from build123d import *

# Parameters (mm, degrees)
BOSS_EXTRUDE2_DEPTH     = 69.85
BOSS_EXTRUDE3_START     = 69.85
BOSS_EXTRUDE3_DEPTH     = 20.6375
BOSS_EXTRUDE4_START     = 90.4875
BOSS_EXTRUDE4_DEPTH     = 23.8125
BOSS_EXTRUDE5_START     = 69.85
BOSS_EXTRUDE5_DEPTH     = 19.05
SKETCH2_R               = 50.8
CUT_EXTRUDE1_DEPTH      = 632.689369865
SKETCH3_R               = 12.7
CUT_EXTRUDE2_DEPTH      = 38.1
CUT_EXTRUDE3_REACH      = 587.992
CUT_EXTRUDE3_END_RADIUS = 73.025
SKETCH4_R               = 7.9375


# Read off the part's stored shape, not the designer's step: Boss-Extrude4
with BuildPart() as part:
    # Sketch1 → Boss-Extrude2 (new body)
    with BuildSketch(Plane(origin=(0, 0, 0), x_dir=(0, 0, -1), z_dir=(1, 0, 0))):
        with BuildLine():
            Line((0, 381), (0, 0))
            Line((0, 0), (-82.55, 0))
            Line((-82.55, 0), (-82.55, -88.9))
            Line((-82.55, -88.9), (69.85, -88.9))
            Line((69.85, -88.9), (69.85, 0))
            Line((69.85, 0), (406.4, 0))
            Line((406.4, 0), (406.4, 117.475))
            Line((406.4, 117.475), (260.35, 117.475))
            Line((260.35, 117.475), (260.35, 111.401610843))
            Line((260.35, 111.401610843), (247.65, 111.401610843))
            Line((247.65, 111.401610843), (247.65, 117.751610843))
            ThreePointArc((247.65, 117.751610843), (181.425166335, 182.404066236), (231.775, 260.060764803))
            Line((231.775, 260.060764803), (231.775, 317.5))
            Line((231.775, 317.5), (76.2, 317.5))
            Line((76.2, 317.5), (76.2, 381))
            Line((76.2, 381), (63.5, 381))
            Line((63.5, 381), (63.5, 368.3))
            Line((63.5, 368.3), (38.1, 368.3))
            Line((38.1, 368.3), (38.1, 381))
            Line((38.1, 381), (0, 381))
        make_face()
    boss_extrude2 = extrude(amount=BOSS_EXTRUDE2_DEPTH)

    # Sketch1<4> → Boss-Extrude3 (add)
    with BuildSketch(Plane(origin=(0, 0, 0), x_dir=(0, 0, -1), z_dir=(1, 0, 0)).offset(BOSS_EXTRUDE3_START)):
        with BuildLine():
            Line((0, 381), (0, 0))
            Line((0, 0), (406.4, 0))
            Line((406.4, 0), (406.4, 190.5))
            ThreePointArc((406.4, 190.5), (388.283807472, 262.566768006), (338.242269675, 317.5))
            Line((338.242269675, 317.5), (76.2, 317.5))
            Line((76.2, 317.5), (76.2, 381))
            Line((76.2, 381), (63.5, 381))
            Line((63.5, 381), (63.5, 368.3))
            Line((63.5, 368.3), (38.1, 368.3))
            Line((38.1, 368.3), (38.1, 381))
            Line((38.1, 381), (0, 381))
        make_face()
        with BuildLine():
            Line((260.35, 117.751610843), (260.35, 111.401610843))
            Line((260.35, 111.401610843), (247.65, 111.401610843))
            Line((247.65, 111.401610843), (247.65, 117.751610843))
            ThreePointArc((247.65, 117.751610843), (254, 263.525), (260.35, 117.751610843))
        make_face(mode=Mode.SUBTRACT)
    boss_extrude3 = extrude(amount=BOSS_EXTRUDE3_DEPTH)

    # Boss-Extrude4 outline → Boss-Extrude4 (add)
    with BuildSketch(Plane(origin=(0, 0, 0), x_dir=(0, 0, -1), z_dir=(1, 0, 0)).offset(BOSS_EXTRUDE4_START)):
        Polygon((406.4, 317.5), (76.2, 317.5), (76.2, 381), (63.5, 381), (63.5, 368.3), (38.1, 368.3), (38.1, 381), (0, 381), (0, 0), (406.4, 0), align=None)
        with BuildLine():
            Line((247.65, 111.401610843), (247.65, 117.751610843))
            ThreePointArc((247.65, 117.751610843), (254, 263.525), (260.35, 117.751610843))
            Line((260.35, 117.751610843), (260.35, 111.401610843))
            Line((260.35, 111.401610843), (247.65, 111.401610843))
        make_face(mode=Mode.SUBTRACT)
    boss_extrude4 = extrude(amount=BOSS_EXTRUDE4_DEPTH)

    # Sketch1<6> → Boss-Extrude5 (add)
    with BuildSketch(Plane(origin=(0, 0, 0), x_dir=(0, 0, -1), z_dir=(1, 0, 0)).offset(BOSS_EXTRUDE5_START)):
        Polygon((69.85, 0), (0, 0), (-82.55, 0), (-82.55, -88.9), (69.85, -88.9), align=None)
    boss_extrude5 = extrude(amount=BOSS_EXTRUDE5_DEPTH)

    # Mirror2: Boss-Extrude2, Boss-Extrude3, Boss-Extrude4, Boss-Extrude5 across plane
    add(boss_extrude2.mirror(Plane(origin=(0, 0, 0), x_dir=(0, 0, 1), z_dir=(1, 0, 0))))
    add(boss_extrude3.mirror(Plane(origin=(0, 0, 0), x_dir=(0, 0, 1), z_dir=(1, 0, 0))))
    add(boss_extrude4.mirror(Plane(origin=(0, 0, 0), x_dir=(0, 0, 1), z_dir=(1, 0, 0))))
    add(boss_extrude5.mirror(Plane(origin=(0, 0, 0), x_dir=(0, 0, 1), z_dir=(1, 0, 0))))

    # Sketch2 → Cut-Extrude1 (cut, through all)
    with BuildSketch(Plane(origin=(0, 381, 0), x_dir=(1, 0, 0), z_dir=(0, 1, 0))):
        with Locations(Location((0, 0, 0), (0, 0, 270))):
            Circle(SKETCH2_R)
        with BuildLine():
            Line((-88.9, -88.9), (88.9, -88.9))
            Line((88.9, -88.9), (88.9, -6.35))
            Line((88.9, -6.35), (87.988181024, -6.35))
            ThreePointArc((87.988181024, -6.35), (83.831130216, -7.899851193), (81.703310951, -11.792857143))
            ThreePointArc((81.703310951, -11.792857143), (0, -82.55), (-81.703310951, -11.792857143))
            ThreePointArc((-81.703310951, -11.792857143), (-83.831130216, -7.899851193), (-87.988181024, -6.35))
            Line((-87.988181024, -6.35), (-88.9, -6.35))
            Line((-88.9, -6.35), (-88.9, -88.9))
        make_face()
    extrude(amount=-CUT_EXTRUDE1_DEPTH, mode=Mode.SUBTRACT)

    # Sketch3 → Cut-Extrude2 (cut)
    with BuildSketch(Plane(origin=(0, 368.3, 0), x_dir=(1, 0, 0), z_dir=(0, 1, 0))):
        with Locations(Location((-79.375, 50.8, 0), (0, 0, 270))):
            Circle(SKETCH3_R)
        with Locations(Location((79.375, 50.8, 0), (0, 0, 270))):
            Circle(SKETCH3_R)
    extrude(amount=-CUT_EXTRUDE2_DEPTH, mode=Mode.SUBTRACT)

    # Cut-Extrude3: up to this cylinder (the profile starts outside it)
    cut_extrude3_end = Plane(origin=(0, 190.5, -254), z_dir=(-1, 0, 0)) * Cylinder(CUT_EXTRUDE3_END_RADIUS, 1508.7715, mode=Mode.PRIVATE)
    # Sketch4 → Cut-Extrude3 (cut, up to the surface)
    with BuildSketch(Plane(origin=(0, 317.5, 0), x_dir=(1, 0, 0), z_dir=(0, 1, 0)), mode=Mode.PRIVATE) as cut_extrude3_sk1:
        with Locations(Location((-92.86875, 254, 0), (0, 0, 270))):
            Circle(SKETCH4_R)
    cut_extrude3_tool1 = extrude(cut_extrude3_sk1.sketch, amount=-CUT_EXTRUDE3_REACH, mode=Mode.PRIVATE) - cut_extrude3_end
    add(cut_extrude3_tool1.solids().sort_by_distance((-92.86875, 317.5, -254))[0], mode=Mode.SUBTRACT)
    # Sketch4 → Cut-Extrude3 (cut, up to the surface)
    with BuildSketch(Plane(origin=(0, 317.5, 0), x_dir=(1, 0, 0), z_dir=(0, 1, 0)), mode=Mode.PRIVATE) as cut_extrude3_sk2:
        with Locations(Location((92.86875, 254, 0), (0, 0, 270))):
            Circle(SKETCH4_R)
    cut_extrude3_tool2 = extrude(cut_extrude3_sk2.sketch, amount=-CUT_EXTRUDE3_REACH, mode=Mode.PRIVATE) - cut_extrude3_end
    add(cut_extrude3_tool2.solids().sort_by_distance((92.86875, 317.5, -254))[0], mode=Mode.SUBTRACT)


solid = part.part
Can you work these out from the model? Positions are in its coordinate system, mm. A direction names the side the tool comes from. Give positions to 0.01 mm unless a question says otherwise; leave off trailing zeros. Loops run counter-clockwise (first coordinate to the right, second up) from the corner with the lowest first, then second, coordinate; pieces in that order, holes last. Notation, with made-up numbers: (64.25, -24.75) - (104.25, -24.75) arc R25 cw to (104.25, -4.75) - close; hole circle Ø9 at (64, 75.5). An arc over 180 degrees is marked (long way). Return JSON: item names as keys, results as strings.
1. I want a section at D-D on x = 43. Please give me the cut outline in (y, z) (3 decimals), and give its area (3 significant figures).
Output values:
{"outline": "(-88.9, -69.85) - (0, -69.85) - (0, -406.4) - (117.475, -406.4) - (117.475, -260.35) - (111.402, -260.35) - (111.402, -247.65) - (117.752, -247.65) arc R73.025 cw to (260.061, -231.775) - (317.5, -231.775) - (317.5, -76.2) - (381, -76.2) - (381, -63.5) - (368.3, -63.5) - (368.3, -38.1) - (381, -38.1) - (381, -27.049) - (-88.9, -27.049) - close; (-88.9, 27.049) - (0, 27.049) - (0, 70.466) - (-88.9, 70.466) - close", "area": "90,700 mm²"}
2. I'm going to push flat-ended pins straight in: pin 1 Ø8 at (x, z) = (65, -99.5) entering from +Y; pin 2 Ø10 at (x, y) = (-5, 237.5) entering from -Z; pin 3 Ø15 at (x, z) = (79.375, -50.8) entering from +Y. Where does each tip first touch, or does it pass through?
Output values:
{"pin 1": "stops at y = 317.5", "pin 2": "stops at z = -202.73", "pin 3": "stops at y = 330.2"}
3. I want a section at A-A on z = -254. Please give me the cut outline in (x, y) (3 decimals), and give its area (3 significant figures).
Output values:
{"outline": "(-114.3, 0) - (114.3, 0) - (114.3, 111.402) - (-114.3, 111.402) - close; (-114.3, 263.525) - (-100.806, 263.525) - (-100.806, 317.5) - (-114.3, 317.5) - close; (-84.931, 263.525) - (-69.85, 263.525) - (-69.85, 317.5) - (-84.931, 317.5) - close; (69.85, 263.525) - (84.931, 263.525) - (84.931, 317.5) - (69.85, 317.5) - close; (100.806, 263.525) - (114.3, 263.525) - (114.3, 317.5) - (100.806, 317.5) - close", "area": "28,600 mm²"}
4. I want a section at C-C on y = 168. Please give me the cut outline in (x, z), and give its area (3 significant figures).
Output values:
{"outline": "(-114.3, -406.4) - (-69.85, -406.4) - (-69.85, -323.47) - (-114.3, -323.47) - close; (-114.3, -184.53) - (114.3, -184.53) - (114.3, 0) - (50.8, 0) arc R50.8 cw to (-50.8, 0) - (-114.3, 0) - close; (69.85, -406.4) - (114.3, -406.4) - (114.3, -323.47) - (69.85, -323.47) - close", "area": "45,500 mm²"}
5. I want a section at B-B on x = 0. Please give me the cut outline in (y, z) (3 decimals), and give its area (3 significant figures).
Output values:
{"outline": "(-88.9, -69.85) - (0, -69.85) - (0, -406.4) - (117.475, -406.4) - (117.475, -260.35) - (111.402, -260.35) - (111.402, -247.65) - (117.752, -247.65) arc R73.025 cw to (260.061, -231.775) - (317.5, -231.775) - (317.5, -76.2) - (381, -76.2) - (381, -63.5) - (368.3, -63.5) - (368.3, -50.8) - (-88.9, -50.8) - close; (-88.9, 50.8) - (0, 50.8) - (0, 82.55) - (-88.9, 82.55) - close", "area": "78,700 mm²"}
6. If I drill on line 1 (X direction, y = 297, z = -254); line 2 (Y direction, x = 38, z = -342) (3 decimals); line 3 (Z direction, x = -91.5, y = 233.5), over which ranges is the centre line in solid material (lowest first)?
Output values:
{"line 1": "x = -114.3 to -100.81, -84.93 to -69.85, 69.85 to 84.93, 100.81 to 114.3", "line 2": "y = 0 to 117.475", "line 3": "z = -406.4 to -313.02, -194.98 to 0"}
7. For faces 1 (the face through (88.9, -44, -31)), 2 (the face through (80, 261.6, -388.8)), 3 (the face through (2, 349, -76.2)), 4 (the face through (-66.783, 349.517, -52.453)), 5 (the face through (-82, 193, 0)), which set-ups out of +Z, -Z, +X, -X, +Y, -Y let a thin tool reach every point of the face, with its end or its side?
Output values:
{"face 1": "+Z, -Z, +X, -Y", "face 2": "-Z, +Y", "face 3": "-Z, +X, -X, +Y", "face 4": "+Y", "face 5": "+Z, +X, -X, +Y"}
8. We'd pull the mould along X, two halves only. Please class faces 6 (the face through (1.65, -43.828, 82.534)), 7 (the face through (75, 375, -38.1)), 8 (the face through (80, 330.2, -51)): +X half, -X half, draft (parallel to the pull), parting line (faces both ways), or undercut.
Output values:
{"face 6": "parting line", "face 7": "draft", "face 8": "undercut"}
